Read the model definition and answer for the solid it produces. Units are mm, in the model's axes. Face numbers are marked on the shaded views. A direction names the side the tool comes from. Give positions to 0.01 mm unless a question says otherwise; leave off trailing zeros. Write each loop counter-clockwise with the first axis right and the second up, starting at its lowest first coordinate (ties: lowest second). Pieces come first, ordered by that corner, then holes. Notation, with made-up numbers: (72, -18) -> (131, -18) arc R18 ccw to (131, 1) -> close; hole circle Ø7 at (18, -39.75). An arc over 180 degrees is marked (long way). Put each result on its own line as item: value. Start each with the question number.
from build123d import *

# Parameters (mm, degrees)
PAD_DEPTH            = 119
THICKNESS_T          = -6
SKETCH001_W          = 300
SKETCH001_H          = 200
POCKET_DEPTH         = 85.001
POCKET_DEPTH_BACK    = -85.001
SKETCH002_R          = 10
SKETCH002_W          = 20
SKETCH002_H          = 20
POCKET001_DEPTH      = 6.001
POCKET001_DEPTH_BACK = -69.001
SKETCH003_R          = 10
POCKET002_DEPTH      = 170.001


with BuildPart() as part:
    # Sketch (on YZ_Plane of Origin) → Pad (new body)
    with BuildSketch(Plane.YZ):
        with BuildLine():
            Line((-85, 75), (85, 75))
            Line((85, 75), (85, 16))
            ThreePointArc((69, 0), (80.313708, 4.686292), (85, 16))
            Line((69, 0), (-69, 0))
            ThreePointArc((-85, 16), (-80.313708, 4.686292), (-69, 0))
            Line((-85, 16), (-85, 75))
        make_face()
    extrude(amount=-PAD_DEPTH)

    # Thickness
    thickness_openings = [part.faces().sort_by_distance(p)[0] for p in [
        (-119, 0, 37.794908),
        (-59.5, 0, 75),
        (0, 0, 37.794908),
    ]]
    offset(amount=THICKNESS_T, openings=thickness_openings)

    # Sketch001 (on XZ_Plane of Origin) → Pocket (cut, two sides)
    with BuildSketch(Plane.XZ) as pocket_sk:
        Rectangle(SKETCH001_W, SKETCH001_H)
        with BuildLine():
            Line((0, 0), (0, 50))
            ThreePointArc((0, 50), (-15.432914, 73.096988), (-42.67767, 67.67767))
            Line((-42.67767, 67.67767), (-89, 21.355339))
            Line((-89, 6), (-89, 21.355339))
            Line((-89, 6), (-119, 6))
            Line((-119, 6), (-119, 0))
            Line((-119, 0), (0, 0))
        make_face(mode=Mode.SUBTRACT)
    extrude(amount=-POCKET_DEPTH, mode=Mode.SUBTRACT)
    extrude(pocket_sk.sketch, amount=-POCKET_DEPTH_BACK, mode=Mode.SUBTRACT)

    # Sketch002 (on Face16 of Pocket) → Pocket001 (cut, two sides)
    with BuildSketch(Plane.XY.offset(6)) as pocket001_sk:
        with Locations((-99, 0)):
            Circle(SKETCH002_R)
        Polygon((-89, 64.820508), (-89, 100), (-169, 100), (-169, -100), (-89, -100), (-89, -64.820508), (-119, -47.5), (-119, 47.5), align=None)
        with Locations((-99, 32)):
            Rectangle(SKETCH002_W, SKETCH002_H)
        with Locations((-99, -32)):
            Rectangle(SKETCH002_W, SKETCH002_H)
    extrude(amount=-POCKET001_DEPTH, mode=Mode.SUBTRACT)
    extrude(pocket001_sk.sketch, amount=-POCKET001_DEPTH_BACK, mode=Mode.SUBTRACT)

    # Sketch003 (on Face14 of Pocket001) → Pocket002 (cut, through all)
    with BuildSketch(Plane.XZ.offset(85)):
        with Locations((-25, 50)):
            Circle(SKETCH003_R)
    extrude(amount=-POCKET002_DEPTH, mode=Mode.SUBTRACT)


solid = part.part
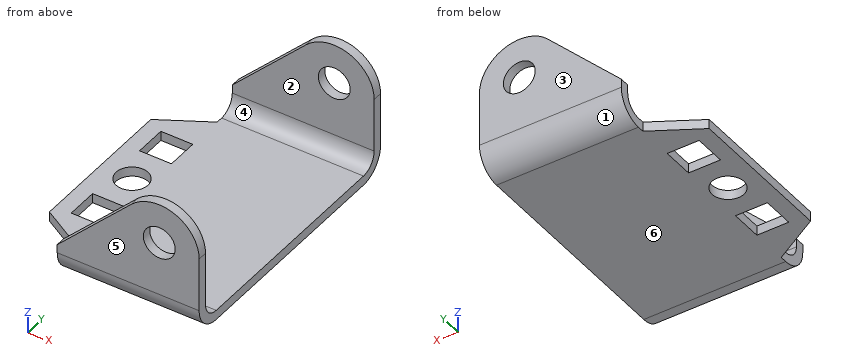
1) A cutting plane is placed at D-D on x = -99. Give the vertices of the cut face in (y, z).
2) For the marked faces 1 and 2, determine the directions among +Z, -Z, +X, -X, +Y, -Y from which every point of the face is accessible in a straight line to the end or side of a thin tool.
3) A cutting plane is placed at A-A on x = -25. Give the vertices of the cut face in (y, z).
4) Each of these flat-tipped pins is pushed along its axis until it touches: pin 1 Ø16 at (x, z) = (-25, 50) entering from +Y; pin 2 Ø5 at (y, z) = (-30, 2) entering from +X; pin 3 Ø6.5 at (x, z) = (-95, 3.5) entering from -Y; pin 4 Ø16 at (y, z) = (77.5, 7) entering from -X. Where does it stop, or does it pass through?
5) Straight lines are drawn through the part: line 1 (Y direction, x = -16, z = 20); line 2 (Z direction, x = -52, y = -59); line 3 (Y direction, x = -60, z = 15). For each, find the intervals that lie inside material, in ascending order. Write a range as [from, to].
6) A cutting plane is placed at B-B on y = 0. Give the vertices of the cut face in (x, z).
7) A cutting plane is placed at C-C on z = 8.5. Give the vertices of the cut face in (x, y), and give its area (3 significant figures).
8) For a pull along Y with two mould halves and no side action, classify the marked faces 3, 4, 5 and 6 as pulls with the +Y half, pulls with the -Y half, needs draft (parallel to the pull), parting line crosses it, or undercut.
Results found:
1. outline: (-59.05, 0) -> (-42, 0) -> (-42, 6) -> (-59.05, 6) -> close; (-22, 0) -> (-10, 0) -> (-10, 6) -> (-22, 6) -> close; (10, 0) -> (22, 0) -> (22, 6) -> (10, 6) -> close; (42, 0) -> (59.05, 0) -> (59.05, 6) -> (42, 6) -> close
2. face 1: -Z, +X, -X, +Y
2. face 2: +Z, +X, -X
3. outline: (-85, 16) arc R16 ccw to (-69, 0) -> (69, 0) arc R16 ccw to (85, 16) -> (85, 40) -> (79, 40) -> (79, 16) arc R10 cw to (69, 6) -> (-69, 6) arc R10 cw to (-79, 16) -> (-79, 40) -> (-85, 40) -> close; (-85, 60) -> (-79, 60) -> (-79, 75) -> (-85, 75) -> close; (79, 60) -> (85, 60) -> (85, 75) -> (79, 75) -> close
4. pin 1: passes through
4. pin 2: stops at x = 0
4. pin 3: stops at y = -63.23
4. pin 4: stops at x = -89
5. line 1: y = [-85, -79], [79, 85]
5. line 2: z = [0, 6]
5. line 3: y = [-84.97, -78.95], [78.95, 84.97]
6. outline: (-119, 0) -> (-109, 0) -> (-109, 6) -> (-119, 6) -> close; (-89, 0) -> (0, 0) -> (0, 6) -> (-89, 6) -> close
7. outline: (-89, -83.13) -> (0, -83.13) -> (0, -75.61) -> (-89, -75.61) -> close; (-89, 75.61) -> (0, 75.61) -> (0, 83.13) -> (-89, 83.13) -> close
7. area: 1,340 mm²
8. face 3: pulls with the +Y half
8. face 4: undercut
8. face 5: pulls with the -Y half
8. face 6: needs draft
